Input: part model. Units: mm. Frame: model coordinates. Give positions to 0.01 mm unless a question says otherwise; leave off trailing zeros. Order: outer loops, then holes, each group sorted by start corner. A loop starts at its lowest first (then second) coordinate and runs counter-clockwise, first axis right, second up. Notation, with made-up numbers: (35, 60.5) -> (41, 60.5) arc R30 cw to (41, 82.5) -> close; hole circle Ø10 at (15.25, -35.5). An arc over 180 degrees is marked (long way). Use a Markdown table: item, result. Add a question column.
from build123d import *

# Parameters (mm, degrees)
F0_R     = 9.5
F1_DEPTH = 10


with BuildPart() as f1:
    # F0 (on Top) → F1 (new body)
    with BuildSketch(Plane.XY):
        Polygon((-155.675, -20), (0, -20), (149.325, -20), (149.325, 20), (0, 20), (-155.675, 20), align=None)
        with Locations((-133.35, 0)):
            Circle(F0_R, mode=Mode.SUBTRACT)
        Circle(F0_R, mode=Mode.SUBTRACT)
        with Locations((127, 0)):
            Circle(F0_R, mode=Mode.SUBTRACT)
    extrude(amount=-F1_DEPTH)


solid = f1.part
Q1. Draft query along X for faces 1 (the flat face through (149.325, 0, -5)), 2 (the flat face through (-5, 9, -10)), 3 (the cylindrical face through (4.38, -8.43, -4.93)). Return one class per face: +X half, -X half, draft (parallel to the pull), parting line (faces both ways), or undercut.
Q2. Ray query, line 1 (X direction, y = -5.5, z = -2) (3 decimals); line 2 (X direction, y = -5, z = -1) (3 decimals); line 3 (Y direction, x = 127, z = -7.25). Return the intervals inside material, ascending.
Q3. Section query C-C (x = -133.35). Return loops of the section in (y, z).
Q4. Section query A-A (y = 0). Return loops of the section in (x, z) (3 decimals).
Q5. Section query B-B (z = -8). Return loops of the section in (x, y) (3 decimals), plus the area to 3 significant figures.
Solution:
| question | item | result |
|---|---|---|
| 1 | face 1 | +X half |
| 1 | face 2 | draft |
| 1 | face 3 | undercut |
| 2 | line 1 | x = -155.675 to -141.096, -125.604 to -7.746, 7.746 to 119.254, 134.746 to 149.325 |
| 2 | line 2 | x = -155.675 to -141.428, -125.272 to -8.078, 8.078 to 118.922, 135.078 to 149.325 |
| 2 | line 3 | y = -20 to -9.5, 9.5 to 20 |
| 3 | outline | (-20, -10) -> (-9.5, -10) -> (-9.5, 0) -> (-20, 0) -> close; (9.5, -10) -> (20, -10) -> (20, 0) -> (9.5, 0) -> close |
| 4 | outline | (-155.675, -10) -> (-142.85, -10) -> (-142.85, 0) -> (-155.675, 0) -> close; (-123.85, -10) -> (-9.5, -10) -> (-9.5, 0) -> (-123.85, 0) -> close; (9.5, -10) -> (117.5, -10) -> (117.5, 0) -> (9.5, 0) -> close; (136.5, -10) -> (149.325, -10) -> (149.325, 0) -> (136.5, 0) -> close |
| 5 | outline | (-155.675, -20) -> (149.325, -20) -> (149.325, 20) -> (-155.675, 20) -> close; hole circle Ø19 at (-133.35, 0); hole circle Ø19 at (0, 0); hole circle Ø19 at (127, 0) |
| 5 | area | 11,300 mm² |
